Can you work these out from the model? Positions are in its coordinate system, mm. Face numbers are marked on the shaded views. A direction names the side the tool comes from. Give positions to 0.01 mm unless a question says otherwise; leave off trailing zeros. Write each loop counter-clockwise with the first axis right and the second up, starting at its lowest first coordinate (ties: lowest second). Pieces come first, ordered by that corner, then holes.
```python
from build123d import *

# Parameters (mm, degrees)
BOSS_EXTRUDE1_DEPTH = 53
SKETCH2_R           = 2.15
CUT_EXTRUDE1_DEPTH  = 40
SKETCH3_R           = 2.55
SKETCH3_R_2         = 2.65
CUT_EXTRUDE2_DEPTH  = 7
FILLET1_R           = 3


with BuildPart() as part:
    # Sketch1 → Boss-Extrude1 (new body)
    with BuildSketch(Plane.XY):
        with BuildLine():
            Line((-9, 45.999997998), (-9, 31.244997998))
            ThreePointArc((-9, 31.244997998), (-4, 33), (1, 31.244997998))
            Line((1, 31.244997998), (1, 45.999997998))
            Line((1, 45.999997998), (-9, 45.999997998))
        make_face()
        with BuildLine():
            ThreePointArc((1, 31.244997998), (-4, 33), (-9, 31.244997998))
            Line((-9, 31.244997998), (1, 31.244997998))
        make_face()
        with BuildLine():
            Line((-8, 18.07179677), (-8, 23.422026616))
            ThreePointArc((-8, 23.422026616), (-4.80311892, 29.224334267), (0.3, 25))
            ThreePointArc((0.3, 25), (0.224334267, 24.19688108), (0, 23.422026616))
            Line((0, 23.422026616), (0, 18.07179677))
            ThreePointArc((0, 18.07179677), (2.92820323, 21), (4, 25))
            ThreePointArc((4, 25), (3.211102551, 28.464101615), (1, 31.244997998))
            Line((1, 31.244997998), (-9, 31.244997998))
            ThreePointArc((-9, 31.244997998), (-11.977048806, 24.394448725), (-8, 18.07179677))
        make_face()
        with BuildLine():
            ThreePointArc((0, 23.422026616), (-1.377907145, 21.591975784), (-3.5, 20.729168699))
            Line((-3.5, 20.729168699), (-3.5, 17.015640289))
            ThreePointArc((-3.5, 17.015640289), (-1.688860318, 17.341107562), (0, 18.07179677))
            Line((0, 18.07179677), (0, 23.422026616))
        make_face()
        with BuildLine():
            ThreePointArc((-4.5, 20.729168699), (-6.622092855, 21.591975784), (-8, 23.422026616))
            Line((-8, 23.422026616), (-8, 18.07179677))
            ThreePointArc((-8, 18.07179677), (-6.311139682, 17.341107562), (-4.5, 17.015640289))
            Line((-4.5, 17.015640289), (-4.5, 20.729168699))
        make_face()
        with BuildLine():
            ThreePointArc((-4.5, 17.015640289), (-6.311139682, 17.341107562), (-8, 18.07179677))
            Line((-8, 18.07179677), (-8, 9))
            Line((-8, 9), (-4.5, 9))
            Line((-4.5, 9), (-4.5, 17.015640289))
        make_face()
        with BuildLine():
            ThreePointArc((0, 18.07179677), (-1.688860318, 17.341107562), (-3.5, 17.015640289))
            Line((-3.5, 17.015640289), (-3.5, 9))
            Line((-3.5, 9), (0, 9))
            Line((0, 9), (0, 18.07179677))
        make_face()
    extrude(amount=BOSS_EXTRUDE1_DEPTH)

    # Sketch2 → Cut-Extrude1 (cut)
    with BuildSketch(Plane(origin=(0, 0, 0), x_dir=(0, 0, -1), z_dir=(1, 0, 0))):
        with Locations((-43, 14)):
            Circle(SKETCH2_R)
        with Locations((-10, 14)):
            Circle(SKETCH2_R)
    extrude(amount=-CUT_EXTRUDE1_DEPTH, mode=Mode.SUBTRACT)

    # Sketch3 → Cut-Extrude2 (cut)
    with BuildSketch(Plane(origin=(0, 45.999997998, 0), x_dir=(1, 0, 0), z_dir=(0, 1, 0))):
        with Locations((-4, -5.5)):
            Circle(SKETCH3_R)
        with Locations((-4, -47.5)):
            Circle(SKETCH3_R_2)
    extrude(amount=-CUT_EXTRUDE2_DEPTH, mode=Mode.SUBTRACT)

    # Fillet1
    fillet1_edges = [part.edges().sort_by_distance(p)[0] for p in [
        (1, 38.622497998, 0),
        (-1.75, 9, 0),
        (-6.25, 9, 0),
        (-9, 38.622497998, 0),
        (-6.25, 9, 53),
        (-1.75, 9, 53),
        (-9, 38.622497998, 53),
        (1, 38.622497998, 53),
    ]]
    fillet(fillet1_edges, radius=FILLET1_R)


solid = part.part
```
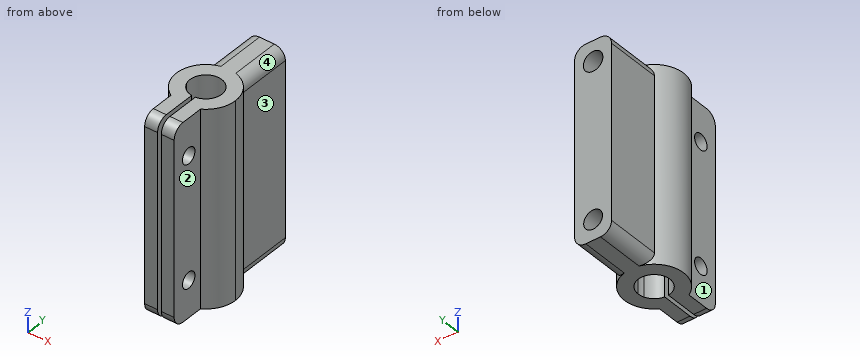
1) Suppose I cut it at B-B on z = 43. Write out the boundary of the cut face in (x, y) (3 decimals).
Values follow:
outline: (-9, 31.245) arc R8 ccw to (-8, 18.072) - (-8, 16.15) - (-4.5, 16.15) - (-4.5, 20.729) arc R4.3 cw (long way) to (-3.5, 20.729) - (-3.5, 16.15) - (0, 16.15) - (0, 18.072) arc R8 ccw to (1, 31.245) - (1, 46) - (-9, 46) - close; (-8, 9) - (-4.5, 9) - (-4.5, 11.85) - (-8, 11.85) - close; (-3.5, 9) - (0, 9) - (0, 11.85) - (-3.5, 11.85) - close
2) Suppose I cut it at C-C on z = 5.5. Write out the boundary of the cut face in (x, y) (3 decimals), plus the area to 3 significant figures.
Values follow:
outline: (-9, 31.245) arc R8 ccw to (-8, 18.072) - (-8, 9) - (-4.5, 9) - (-4.5, 20.729) arc R4.3 cw (long way) to (-3.5, 20.729) - (-3.5, 9) - (0, 9) - (0, 18.072) arc R8 ccw to (1, 31.245) - (1, 46) - (-1.45, 46) - (-1.45, 39) - (-6.55, 39) - (-6.55, 46) - (-9, 46) - close
area: 298 mm2
3) Suppose I cut it at D-D on z = 14.5. Write out the boundary of the cut face in (x, y) (3 decimals), plus the area to 3 significant figures.
Values follow:
outline: (-9, 31.245) arc R8 ccw to (-8, 18.072) - (-8, 9) - (-4.5, 9) - (-4.5, 20.729) arc R4.3 cw (long way) to (-3.5, 20.729) - (-3.5, 9) - (0, 9) - (0, 18.072) arc R8 ccw to (1, 31.245) - (1, 46) - (-9, 46) - close
area: 334 mm2
4) For the marked faces 1, 2, 3 and 4, which set-ups out of +Z, -Z, +X, -X, +Y, -Y let a thin tool reach every point of the face, with its end or its side?
Values follow:
face 1: +Z, -Z, -X, -Y
face 2: +Z, -Z, +X, -Y
face 3: +Z, -Z, +X, +Y
face 4: +Z, +X, +Y
5) For pin 1 Ø6 at (y, z) = (15.5, 21) entering from +X; pin 2 Ø2 at (y, z) = (38.5, 32) entering from -X; pin 3 Ø4 at (y, z) = (14, 43) entering from -X; pin 4 Ø1.6 at (x, z) = (-3, 49) entering from +Y, each with a flat end and sliding along its axis, tell me the tip position at first contact or that it passes through.
Values follow:
pin 1: stops at x = 0.66
pin 2: stops at x = -9
pin 3: passes through
pin 4: stops at y = 39
6) Suppose I cut it at A-A on y = 17.5. Write out the boundary of the cut face in (x, z), plus the area to 3 significant figures.
Values follow:
outline: (-8, 0) - (-4.5, 0) - (-4.5, 53) - (-8, 53) - close; (-3.5, 0) - (0, 0) - (0, 53) - (-3.5, 53) - close
area: 371 mm2
7) Please list where these lines run through material, in increasing order: L1, parallel to X at y = 17, z = 10.5; L2, parallel to Y at x = -6.3, z = 10; L3, parallel to Y at x = -1, z = 10.
Values follow:
L1: x = -8 to -4.5, -3.5 to 0
L2: y = 9 to 11.85, 16.15 to 21.37, 28.63 to 46
L3: y = 9 to 11.85, 16.15 to 21.92, 28.08 to 46
